Autodesk Inventor part; units mm, degrees
ref_plane "Work Plane2" through (0, 0, 0.4) normal (0, 0, -1) x (-1, 0, 0)
ref_plane "YZ Plane" through (0, 0, 0) normal (1, 0, 0) x (0, 1, 0)
ref_plane "XZ Plane" through (0, 0, 0) normal (0, 1, 0) x (-1, 0, 0)
sketch "Sketch1" plane through (0, 0, 0) normal (0, 0, 1) x (1, 0, 0)
  line L0 (6.0134, 0.5413) -> (-66.0587, 0.5413)
  circle A0 centre (-66.0587, 68.5413) radius 8 construction
  line L1 (-66.0587, 60.5413) -> (6.0134, 60.5413) construction
  line L2 (-66.0587, 76.5413) -> (-58.0587, 68.5413)
  line L3 (-66.0587, 60.5413) -> (-58.0587, 68.5413)
  line L4 (6.0134, 60.5413) -> (6.0134, 0.5413)
  line L5 (-66.0587, 0.5413) -> (-66.0587, 60.5413)
  line L6 (-66.0587, 76.5413) -> (-66.0587, 80.5413)
  line L7 (6.0134, 0.5413) -> (-120, 0.5413) construction
  line L8 (-60, 0) -> (-60, 75) construction
  line L9 (-60, 75) -> (0, 75) construction
  line L10 (6.0134, 150.5413) -> (6.0134, 0.5413) construction
  line L11 (6.0134, 60.5413) -> (6.0134, 80.5413)
  line L12 (-66.0587, 80.5413) -> (6.0134, 80.5413)
  line L13 (-66.0587, 76.5413) -> (12.8048, 76.5413) construction
  line L14 (-58.0587, 68.5413) -> (17.3629, 68.5413) construction
  line L15 (-66.0587, 60.5413) -> (24.3855, 60.5413) construction
  circle A1 centre (6.0134, 68.5413) radius 8 construction
  line L16 (6.0134, 60.5413) -> (14.0134, 68.5413)
  line L17 (14.0134, 68.5413) -> (6.0134, 76.5413)
  point P0 (0, 0)
  dimension "d1" = 80
  dimension "d5" = 16
  dimension "d6" = 60
extrude "Extrusion1" add sketch "Sketch1" along normal blind 4
sketch "Sketch3" plane through (0, 0, 4) normal (0, 0, 1) x (1, 0, 0)
  line L0 (-66.0587, 80.5413) -> (13.9413, 80.5413) construction
  line L1 (-34.8487, 75.4475) -> (-28.5043, 75.4475) construction
  line L2 (-28.5043, 75.4475) -> (-28.5043, 84.7097) construction
  line L3 (-28.5043, 84.7097) -> (-34.8487, 84.7097) construction
  line L4 (-34.8487, 84.7097) -> (-34.8487, 75.4475) construction
  line L5 (-52.9694, 57.7889) -> (-12.0353, 57.7889)
  line L6 (-12.0353, 57.7889) -> (-12.0353, 60.7889)
  line L7 (-12.0353, 60.7889) -> (-3.3751, 55.7889)
  line L8 (-12.0353, 50.7889) -> (-3.3751, 55.7889)
  line L9 (-12.0353, 50.7889) -> (-12.0353, 53.7889)
  line L10 (-52.9694, 53.7889) -> (-12.0353, 53.7889)
  line L11 (-52.9694, 57.7889) -> (-52.9694, 53.7889)
  line L12 (-27, 50.7889) -> (-31, 50.7889)
  line L13 (-31, 50.7889) -> (-31, 46.7889)
  line L14 (-27, 46.7889) -> (-27, 50.7889)
  line L15 (-27, 50.7889) -> (-27, 52.7889) construction
  line L16 (-27, 35.7889) -> (-27, 32.7889) construction
  line L17 (-27, 32.7889) -> (-33, 32.7889)
  line L18 (-33, 32.7889) -> (-33, 28.7889)
  line L19 (-33, 28.7889) -> (-27, 28.7889)
  line L20 (-27, 28.7889) -> (-27, 32.7889)
  line L21 (-33, 32.7889) -> (-36, 32.7889) construction
  line L22 (-36, 32.7889) -> (-36, 28.7889)
  line L23 (-36, 32.7889) -> (-42.4587, 32.7889)
  line L24 (-42.4587, 32.7889) -> (-42.4587, 35.7889)
  line L25 (-42.4587, 35.7889) -> (-51.0587, 30.7889)
  line L26 (-36, 28.7889) -> (-42.4587, 28.7889)
  line L27 (-42.4587, 28.7889) -> (-42.4587, 25.7889)
  line L28 (-42.4587, 25.7889) -> (-51.0587, 30.7889)
  line L29 (6.0134, 0.5413) -> (-66.0587, 0.5413) construction
  line L30 (-66.0587, 80.5413) -> (6.0134, 80.5413) construction
  line L31 (-30.0226, 80.5413) -> (-30.0226, 0.5413) construction
  line L32 (-24, 32.7889) -> (-18, 32.7889)
  line L33 (-18, 32.7889) -> (-18, 28.7889)
  line L34 (-18, 28.7889) -> (-24, 28.7889)
  line L35 (-24, 28.7889) -> (-24, 32.7889)
  line L36 (-15, 32.7889) -> (-9, 32.7889)
  line L37 (-9, 32.7889) -> (-9, 28.7889)
  line L38 (-9, 28.7889) -> (-15, 28.7889)
  line L39 (-15, 28.7889) -> (-15, 32.7889)
  line L40 (-27, 46.7889) -> (-24, 46.7889)
  line L41 (-31, 46.7889) -> (-34, 46.7889)
  line L42 (-66.0587, 0.5413) -> (-66.0587, 60.5413) construction
  line L43 (6.0134, 60.5413) -> (6.0134, 0.5413) construction
  line L44 (-29, 50.7889) -> (-29, 38.1889) construction
  line L45 (-34, 46.7889) -> (-29, 38.1889)
  line L46 (-24, 46.7889) -> (-29, 38.1889)
  line L47 (-24.1712, 63.2475) -> (-26.277, 63.2475)
  line L48 (-26.277, 63.2475) -> (-30.1328, 68.1018)
  line L49 (-30.1328, 68.1018) -> (-31.9915, 68.1018)
  line L50 (-31.9915, 68.1018) -> (-31.9915, 63.2475)
  line L51 (-31.9915, 63.2475) -> (-33.6129, 63.2475)
  line L52 (-33.6129, 63.2475) -> (-33.6129, 75.4475)
  line L53 (-33.6129, 75.4475) -> (-30.4689, 75.4475)
  spline S0 degree 2 poles (-30.4689, 75.4475) (-29.421, 75.4475) (-28.0072, 75.2201) (-27.3646, 74.8048) knots 0 0 0 1 2 2 2
  spline S1 degree 2 poles (-27.3646, 74.8048) (-26.7219, 74.3896) (-25.9804, 73.0945) (-25.9804, 72.1355) knots 0 0 0 1 2 2 2
  spline S2 degree 2 poles (-25.9804, 72.1355) (-25.9804, 70.8008) (-27.3448, 68.9915) (-28.5114, 68.5565) knots 0 0 0 1 2 2 2
  line L54 (-28.5114, 68.5565) -> (-24.1712, 63.2475)
  spline S3 degree 2 poles (-27.671, 72.0069) (-27.671, 72.5408) (-28.0467, 73.3614) (-28.4422, 73.6283) knots 0 0 0 1 2 2 2
  spline S4 degree 2 poles (-28.4422, 73.6283) (-28.7882, 73.8557) (-29.7077, 74.0436) (-30.38, 74.0436) knots 0 0 0 1 2 2 2
  line L55 (-30.38, 74.0436) -> (-31.9915, 74.0436)
  line L56 (-31.9915, 74.0436) -> (-31.9915, 69.4562)
  line L57 (-31.9915, 69.4562) -> (-30.5678, 69.4562)
  spline S5 degree 2 poles (-30.5678, 69.4562) (-29.8659, 69.4562) (-28.7487, 69.7034) (-28.3631, 70.089) knots 0 0 0 1 2 2 2
  spline S6 degree 2 poles (-28.3631, 70.089) (-28.0072, 70.4251) (-27.671, 71.3742) (-27.671, 72.0069) knots 0 0 0 1 2 2 2
  point P0 (-26.0587, 80.5413)
  point P1 (-12.0353, 60.7889)
  point P2 (-42.4587, 34.2889)
  point P3 (6.0134, 30.5413)
  point P4 (-9, 30.7889)
  point P5 (-25.5, 46.7889)
  dimension "d65" = 4
  dimension "d66" = 3
  dimension "d67" = 10
  dimension "d68" = 3
  dimension "d88" = 4
  dimension "d92" = 6
  dimension "d93" = 4
  dimension "d94" = 3
  dimension "d96" = 3
  dimension "d97" = 3
  dimension "d121" = 6
  dimension "d122" = 4
  dimension "d123" = 6
  dimension "d124" = 3
  dimension "d125" = 3
  dimension "d128" = 3
  dimension "d130" = 4
  dimension "d132" = 3
  dimension "d133" = 3
  dimension "d134" = 8.6
  dimension "d135" = 15
  dimension "d136" = 15.0134
  dimension "d137" = 12.6
  dimension "d138" = 4
extrude "Extrusion3" cut sketch "Sketch3" against normal blind 1.5
ref_plane "Work Plane2" through (0, 0, 0.4) normal (0, 0, -1) x (-1, 0, 0)
sketch "Sketch5" plane through (0, 0, 0.4) normal (0, 0, -1) x (-1, 0, 0)
  line L0 (-13.9413, 80.5413) -> (66.0587, 80.5413) construction
  line L1 (-6.0134, 0.5413) -> (-6.0134, 76.5413) construction
  line L2 (66.0587, 0.5413) -> (-6.0134, 0.5413) construction
  line L3 (66.0587, 60.5413) -> (66.0587, 0.5413) construction
  line L4 (66.0587, 80.5413) -> (66.0587, 76.5413) construction
  line L5 (-6.0134, 0.5413) -> (-6.0134, 60.5413) construction
  line L6 (66.0587, 0.5413) -> (-6.0134, 0.5413) construction
  line L7 (66.0587, 60.5413) -> (66.0587, 0.5413) construction
  line L8 (58.0587, 68.5413) -> (66.0587, 60.5413) construction
  line L9 (66.0587, 76.5413) -> (58.0587, 68.5413) construction
  circle A0 centre (30.0226, 14.5413) radius 3.075
  line L10 (31, 46.7889) -> (31, 50.7889) construction
  line L11 (31, 50.7889) -> (27, 50.7889) construction
  line L12 (27, 50.7889) -> (27, 46.7889) construction
  line L13 (3.3751, 55.7889) -> (12.0353, 50.7889) construction
  line L14 (12.0353, 50.7889) -> (12.0353, 53.7889) construction
  line L15 (12.0353, 53.7889) -> (52.9694, 53.7889) construction
  line L16 (52.9694, 53.7889) -> (52.9694, 57.7889) construction
  line L17 (52.9694, 57.7889) -> (12.0353, 57.7889) construction
  line L18 (12.0353, 57.7889) -> (12.0353, 60.7889) construction
  line L19 (12.0353, 60.7889) -> (3.3751, 55.7889) construction
  line L20 (42.4587, 25.7889) -> (51.0587, 30.7889) construction
  line L21 (51.0587, 30.7889) -> (42.4587, 35.7889) construction
  line L22 (42.4587, 35.7889) -> (42.4587, 32.7889) construction
  line L23 (42.4587, 32.7889) -> (36, 32.7889) construction
  line L24 (36, 32.7889) -> (36, 28.7889) construction
  line L25 (36, 28.7889) -> (42.4587, 28.7889) construction
  line L26 (42.4587, 28.7889) -> (42.4587, 25.7889) construction
  line L27 (27, 28.7889) -> (33, 28.7889) construction
  line L28 (33, 28.7889) -> (33, 32.7889) construction
  line L29 (33, 32.7889) -> (27, 32.7889) construction
  line L30 (27, 32.7889) -> (27, 28.7889) construction
  line L31 (66.0587, 76.5413) -> (66.0587, 80.5413) construction
  line L32 (58.0587, 68.5413) -> (66.0587, 76.5413) construction
  line L33 (66.0587, 60.5413) -> (58.0587, 68.5413) construction
  line L34 (66.0587, 0.5413) -> (66.0587, 60.5413) construction
  line L35 (-6.0134, 0.5413) -> (66.0587, 0.5413) construction
  line L36 (-6.0134, 60.5413) -> (-6.0134, 0.5413) construction
  line L37 (-6.0134, 80.5413) -> (66.0587, 80.5413)
  line L38 (66.0587, 80.5413) -> (-6.0134, 80.5413)
  line L39 (-6.0134, 76.5413) -> (-6.0134, 80.5413)
  line L40 (-14.0134, 68.5413) -> (-6.0134, 76.5413)
  line L41 (-6.0134, 60.5413) -> (-14.0134, 68.5413)
  line L42 (-14.0134, 68.5413) -> (-6.0134, 60.5413)
  line L43 (-6.0134, 76.5413) -> (-14.0134, 68.5413)
  line L44 (-6.0134, 80.5413) -> (-6.0134, 76.5413)
  line L45 (27, 46.7889) -> (24, 46.7889)
  line L46 (24, 46.7889) -> (29, 38.1889)
  line L47 (29, 38.1889) -> (34, 46.7889)
  line L48 (34, 46.7889) -> (31, 46.7889)
  dimension "d99" = 80
  dimension "d100" = 72.0721
  dimension "d101" = 6.15
  dimension "d102" = 14
  dimension "d103" = 36.036
extrude "Extrusion4" cut sketch "Sketch5" against normal blind 3.15
sketch "Sketch7" plane through (0, 0, 4) normal (0, 0, 1) x (1, 0, 0)
  line L0 (-66.0587, 0.5413) -> (-66.0587, 60.5413) construction
  line L1 (6.0134, 0.5413) -> (-66.0587, 0.5413) construction
  line L2 (6.0134, 80.5413) -> (6.0134, 0.5413) construction
  line L3 (-58.2371, 23.7889) -> (9.8349, 23.7889)
  line L4 (6.0134, 2.5413) -> (-64.0587, 2.5413)
  line L5 (7.8349, 22.5889) -> (-56.2371, 22.5889)
  line L6 (-62.0587, 3.7413) -> (2.0134, 3.7413)
  line L7 (-56.2371, 22.5889) -> (-58.2371, 22.5889)
  line L8 (7.8349, 22.5889) -> (9.8349, 22.5889)
  line L9 (2.0134, 3.7413) -> (4.0134, 3.7413)
  line L10 (-62.0587, 3.7413) -> (-64.0587, 3.7413)
  line L11 (-58.2371, 23.7889) -> (-66.0587, 23.7889)
  line L12 (-58.2371, 22.5889) -> (-66.0587, 22.5889)
  line L13 (-66.0587, 23.7889) -> (-66.0587, 22.5889)
  line L14 (-64.0587, 3.7413) -> (-66.0587, 3.7413)
  line L15 (-64.0587, 2.5413) -> (-66.0587, 2.5413)
  line L16 (-66.0587, 3.7413) -> (-66.0587, 2.5413)
  line L17 (9.8349, 23.7889) -> (6.0134, 23.7889)
  line L18 (9.8349, 22.5889) -> (6.0134, 22.5889)
  line L19 (6.0134, 23.7889) -> (6.0134, 22.5889)
  line L20 (4.0134, 3.7413) -> (6.0134, 3.7413)
  line L21 (6.0134, 3.7413) -> (6.0134, 2.5413)
  point P0 (-42.4587, 25.7889)
  point P1 (6.0134, 60.5413)
  point P2 (0, 0)
  dimension "d115" = 2
  dimension "d116" = 2
  dimension "d117" = 1.2
  dimension "d120" = 1.2
extrude "Extrusion5" cut sketch "Sketch7" against normal blind 0.2
sketch "Sketch8" plane through (-66.0587, 0.5413, 0) normal (0, -1, 0) x (1, 0, 0)
  line L0 (72.0721, 4) -> (0, 4) construction
  line L1 (0, 0) -> (0, 4) construction
  line L2 (0, 0) -> (72.0721, 0) construction
  line L3 (72.0721, 0) -> (72.0721, 4) construction
  line L4 (72.0721, 4) -> (0, 4) construction
  line L5 (0, 0) -> (0, 4) construction
  line L6 (0, 0) -> (72.0721, 0) construction
  line L7 (72.0721, 0) -> (72.0721, 4) construction
  point P0 (66.0587, 0)
properties part number "MS_R[203] text 80x60"
Model file for the job. Use its own axes, mm. A direction names the side the tool comes from. Coordinates: 2 decimals unless noted, no trailing zeros. Loops run counter-clockwise (first coordinate to the right, second up) from the corner with the lowest first, then second, coordinate; pieces in that order, holes last. Notation, with made-up numbers: (31.25, 16.5) -> (79.25, 16.5) arc R17 ccw to (79.25, 46.5) -> close; hole circle Ø2 at (-37, 71). An arc over 180 degrees is marked (long way). Use one line per item in the form item = value. Start each with the question number.
(1) Tool access for faces 5 (the flat face through (-30, 15, 3.55)), 6 (the flat face through (-46.699, 33.324, 3.26)), 7 (the flat face through (6.013, 31, 2)), 8 (the flat face through (-62.115, 72.597, 1.972)), 9 (the flat face through (-27, 41, 0)): list every direction of +Z, -Z, +X, -X, +Y, -Y with a clear straight run to the whole face (end or side of a thin tool).
(2) Cut at A-A on x = -52. Give the cut face in (y, z).
(3) Cut at B-B on y = 37. Give the cut face in (x, z), and give its area (3 significant figures).
(4) Pull direction Y, two halves, no side cores. Call faces 1 (the flat face through (-7.766, 58.324, 3.26)), 2 (the flat face through (9.96, 64.49, 1.97)), 3 (the flat face through (-27, 53, 4)), 4 (the flat face through (-26.465, 42.549, 3.26)): pulls with the +Y half, pulls with the -Y half, needs draft (parallel to the pull), parting line crosses it, or undercut.
(5) Probe probe 1 along Y at (x, z) = (-23.5, 2.75); probe 2 along X at (y, z) = (31.5, 3.75); probe 3 along X at (y, z) = (6, 1.45). List the from-to ranges inside material, lowest first. Write a range as from..to.
(6) Flat gauge pins, fed straight in: pin 1 (1.2 mm diameter, centred on x = -21.5, y = 31.5, fed in from +Z); pin 2 (1.2 mm diameter, centred on y = 72, z = 3, fed in from -X). Where does each tip first touch, or does it go through?
Values:
q1.face_5 = none
q1.face_6 = +Z
q1.face_7 = +Z, -Z, +X, -Y
q1.face_8 = +Z, -Z, -X
q1.face_9 = -Z, +X, -X, +Y, -Y
q2.outline = (0.54, 0) -> (80.54, 0) -> (80.54, 4) -> (57.79, 4) -> (57.79, 2.5) -> (53.79, 2.5) -> (53.79, 4) -> (23.79, 4) -> (23.79, 3.8) -> (22.59, 3.8) -> (22.59, 4) -> (3.74, 4) -> (3.74, 3.8) -> (2.54, 3.8) -> (2.54, 4) -> (0.54, 4) -> close
q3.outline = (-66.06, 0) -> (6.01, 0) -> (6.01, 4) -> (-66.06, 4) -> close
q3.area = 288 mm2
q4.face_1 = undercut
q4.face_2 = pulls with the -Y half
q4.face_3 = needs draft
q4.face_4 = undercut
q5.probe_1 = 0.54..28.79, 32.79..53.79, 57.79..80.54
q5.probe_2 = -66.06..-49.84, -36..-33, -27..-24, -18..-15, -9..6.01
q5.probe_3 = -66.06..6.01
q6.pin_1 = 2.5
q6.pin_2 = -62.12
